Study the drawing (mm; zero at the part's minimum x, y, z) and answer. Round coordinates to 2 decimals unless told otherwise and drop trailing zeros. Order: outer loops, then holes, each group sorted by start corner. A loop starts at its lowest first (then second) coordinate and runs counter-clockwise, first axis right, second up. Notation, with made-up numbers: M 59.5,64 L 104.5,64 A30 ccw 104.5,96 Z; hole C 55.25,21 d5. An arc over 180 degrees is marked long. Put each result on its own line as item: value. Start each with the question number.
1. The part is cut by section B-B (x = 7). Give the vertices of the cut face in (y, z).
2. The part is cut by section D-D (z = 9). Give the vertices of the cut face in (x, y).
3. The mould has two halves that part along X. Classify the marked faces 1, 2, 3 and 4: +X half, -X half, draft (parallel to the pull), parting line (faces both ways), or undercut.
4. The part is cut by section A-A (y = 4.3). Give the vertices of the cut face in (x, z).
5. Consider line 1 (X direction, y = 2.75, z = 5); line 2 (X direction, y = 2.2, z = 4.5) (1 decimal); line 3 (Z direction, x = 3.5, y = 1.75). Determine where each line is inside the solid, lowest interval first.
6. The part is cut by section C-C (y = 3.25). Give the vertices of the cut face in (x, z).
7. Each of these flat-tipped pins is pushed along its axis until it touches: pin 1 Ø1 at (x, z) = (7, 7) entering from -Y; pin 2 Ø5.5 at (x, z) = (6.5, 3.5) entering from -Y; pin 3 Ø1.5 at (y, z) = (3.5, 6.5) entering from +X. Where does it stop, or does it pass through?
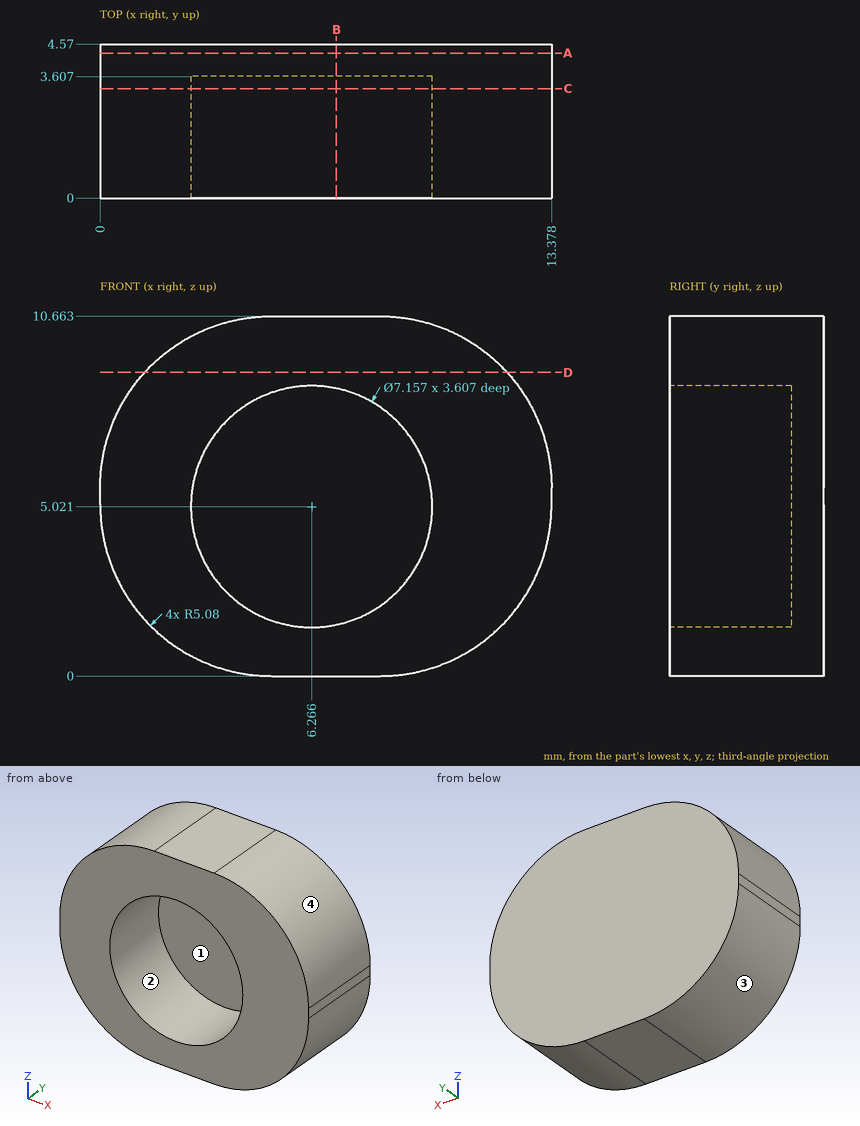
Resolved:
1. outline: M 0,0 L 4.57,0 L 4.57,10.66 L 0,10.66 L 0,8.52 L 3.61,8.52 L 3.61,1.52 L 0,1.52 Z
2. outline: M 1.32,0 L 12.06,0 L 12.06,4.57 L 1.32,4.57 Z
3. face 1: undercut
3. face 2: undercut
3. face 3: -X half
3. face 4: +X half
4. outline: M 0,5.08 A5.08 ccw 5.08,0 L 8.3,0 A5.08 ccw 13.38,5.08 L 13.38,5.58 A5.08 ccw 8.3,10.66 L 5.08,10.66 A5.08 ccw 0,5.58 Z
5. line 1: 0 to 2.69, 9.84 to 13.38
5. line 2: 0 to 2.7, 9.8 to 13.3
5. line 3: 0.25 to 2.75, 7.29 to 10.41
6. outline: M 0,5.08 A5.08 ccw 5.08,0 L 8.3,0 A5.08 ccw 13.38,5.08 L 13.38,5.58 A5.08 ccw 8.3,10.66 L 5.08,10.66 A5.08 ccw 0,5.58 Z; hole C 6.27,5.02 d7.16
7. pin 1: y = 3.61
7. pin 2: y = 0
7. pin 3: x = 13.38
